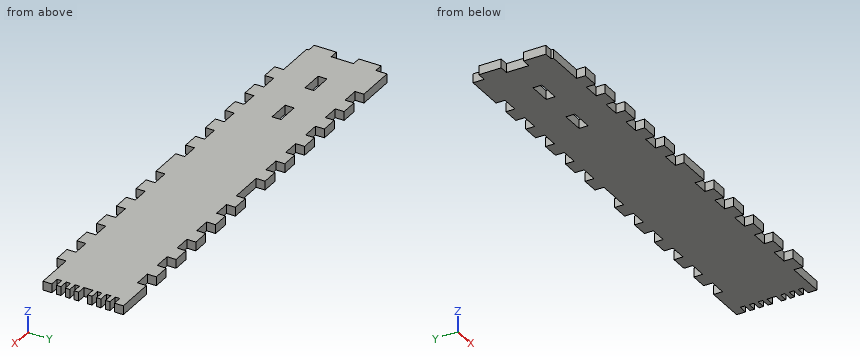
from build123d import *

# Parameters (mm, degrees)
ESQUISSE1_W             = 400
ESQUISSE1_H             = 80
BOSS_EXTRU_1_DEPTH      = 8
ESQUISSE2_W             = 8
ESQUISSE2_H             = 20
BOSS_EXTRU_2_DEPTH      = 8
ESQUISSE4_W             = 15
ESQUISSE4_H             = 8
ENL_V_MAT_EXTRU_1_DEPTH = 212.962260792
ESQUISSE5_W             = 15
ESQUISSE5_H             = 8
ESQUISSE5_W_2           = 35
ENL_V_MAT_EXTRU_2_DEPTH = 212.962260792
ESQUISSE6_W             = 20
ESQUISSE6_H             = 8
ENL_V_MAT_EXTRU_3_DEPTH = 212.962260792
ESQUISSE8_W             = 8
ESQUISSE8_H             = 4
ENL_V_MAT_EXTRU_5_DEPTH = 212.962260792


with BuildPart() as part:
    # Esquisse1 → Boss.-Extru.1 (new body)
    with BuildSketch(Plane.XY):
        Rectangle(ESQUISSE1_W, ESQUISSE1_H)
    extrude(amount=BOSS_EXTRU_1_DEPTH)

    # Esquisse2 → Boss.-Extru.2 (add)
    with BuildSketch(Plane.XY):
        with Locations((-204, 20)):
            Rectangle(ESQUISSE2_W, ESQUISSE2_H)
        with Locations((-204, -20)):
            Rectangle(ESQUISSE2_W, ESQUISSE2_H)
    extrude(amount=BOSS_EXTRU_2_DEPTH)

    # Esquisse4 → Enlèv. mat.-Extru.1 (cut, through all)
    with BuildSketch(Plane.XY):
        Polygon((0, 40), (-15, 40), (-15, 32), (0, 32), (15, 32), (15, 40), align=None)
        with Locations((-37.5, 36)):
            Rectangle(ESQUISSE4_W, ESQUISSE4_H)
        with Locations((-67.5, 36)):
            Rectangle(ESQUISSE4_W, ESQUISSE4_H)
        with Locations((-97.5, 36)):
            Rectangle(ESQUISSE4_W, ESQUISSE4_H)
        with Locations((-127.5, 36)):
            Rectangle(ESQUISSE4_W, ESQUISSE4_H)
        with Locations((-157.5, 36)):
            Rectangle(ESQUISSE4_W, ESQUISSE4_H)
        with Locations((37.5, 36)):
            Rectangle(ESQUISSE4_W, ESQUISSE4_H)
        with Locations((67.5, 36)):
            Rectangle(ESQUISSE4_W, ESQUISSE4_H)
        with Locations((97.5, 36)):
            Rectangle(ESQUISSE4_W, ESQUISSE4_H)
        with Locations((127.5, 36)):
            Rectangle(ESQUISSE4_W, ESQUISSE4_H)
        with Locations((157.5, 36)):
            Rectangle(ESQUISSE4_W, ESQUISSE4_H)
    extrude(amount=ENL_V_MAT_EXTRU_1_DEPTH, mode=Mode.SUBTRACT)

    # Esquisse5 → Enlèv. mat.-Extru.2 (cut, through all)
    with BuildSketch(Plane.XY):
        with Locations((-22.5, -36)):
            Rectangle(ESQUISSE5_W, ESQUISSE5_H)
        with Locations((-52.5, -36)):
            Rectangle(ESQUISSE5_W, ESQUISSE5_H)
        with Locations((-82.5, -36)):
            Rectangle(ESQUISSE5_W, ESQUISSE5_H)
        with Locations((-112.5, -36)):
            Rectangle(ESQUISSE5_W, ESQUISSE5_H)
        with Locations((-142.5, -36)):
            Rectangle(ESQUISSE5_W, ESQUISSE5_H)
        with Locations((-182.5, -36)):
            Rectangle(ESQUISSE5_W_2, ESQUISSE5_H)
        with Locations((22.5, -36)):
            Rectangle(ESQUISSE5_W, ESQUISSE5_H)
        with Locations((52.5, -36)):
            Rectangle(ESQUISSE5_W, ESQUISSE5_H)
        with Locations((82.5, -36)):
            Rectangle(ESQUISSE5_W, ESQUISSE5_H)
        with Locations((112.5, -36)):
            Rectangle(ESQUISSE5_W, ESQUISSE5_H)
        with Locations((142.5, -36)):
            Rectangle(ESQUISSE5_W, ESQUISSE5_H)
        with Locations((182.5, -36)):
            Rectangle(ESQUISSE5_W_2, ESQUISSE5_H)
    extrude(amount=ENL_V_MAT_EXTRU_2_DEPTH, mode=Mode.SUBTRACT)

    # Esquisse6 → Enlèv. mat.-Extru.3 (cut, through all)
    with BuildSketch(Plane.XY):
        with Locations((-160, 0)):
            Rectangle(ESQUISSE6_W, ESQUISSE6_H)
        with Locations((-110, 0)):
            Rectangle(ESQUISSE6_W, ESQUISSE6_H)
    extrude(amount=ENL_V_MAT_EXTRU_3_DEPTH, mode=Mode.SUBTRACT)

    # Esquisse8 → Enlèv. mat.-Extru.5 (cut, through all)
    with BuildSketch(Plane.XY):
        Polygon((200, 4), (200, 8), (192, 8), (192, 4), (192, 0), (200, 0), align=None)
        with Locations((196, 14)):
            Rectangle(ESQUISSE8_W, ESQUISSE8_H)
        with Locations((196, 22)):
            Rectangle(ESQUISSE8_W, ESQUISSE8_H)
        with Locations((196, 30)):
            Rectangle(ESQUISSE8_W, ESQUISSE8_H)
        with Locations((196, -6)):
            Rectangle(ESQUISSE8_W, ESQUISSE8_H)
        with Locations((196, -14)):
            Rectangle(ESQUISSE8_W, ESQUISSE8_H)
        with Locations((196, -22)):
            Rectangle(ESQUISSE8_W, ESQUISSE8_H)
    extrude(amount=ENL_V_MAT_EXTRU_5_DEPTH, mode=Mode.SUBTRACT)


solid = part.part
Model file for the job. Use its own axes, mm. Give positions to 0.01 mm unless a question says otherwise; leave off trailing zeros. Loops run counter-clockwise (first coordinate to the right, second up) from the corner with the lowest first, then second, coordinate; pieces in that order, holes last. Notation, with made-up numbers: (89.5, -5.75) - (145.5, -5.75) arc R22 cw to (145.5, 18.25) - close; hole circle Ø3 at (-19, -7). An arc over 180 degrees is marked (long way). Use one line per item in the form item = value.
(1) Cut at B-B (z = 6). Count the separate pieces of the cut face and the enclosed holes in it, then the cut area to 3 significant figures.
Determined:
separate_pieces = 1
enclosed_holes = 2
area = 28,500 mm^2
(2) Drill centre lines: L1, parallel to X at y = 5, z = 1; L2, parallel to Y at x = 27, z = 5; L3, parallel to Y at x = -157, z = 7.75. Where is each one in solid material? Low to high.
Determined:
L1 = -200 to 192
L2 = -32 to 40
L3 = -40 to -4, 4 to 32
(3) Drop flat-ended pins along their axis: P1, Ø1, axis at x = -129, z = 6, coming from the +Y side; P2, Ø1.5, axis at x = 112, z = 6, coming from the -Y side; P3, Ø3, axis at y = 5.5, z = 5.5, coming from the +X side; P4, Ø5, axis at x = 73, y = -22, coming from the -Z side. Give the stop position or say it passes through.
Determined:
P1 = 32
P2 = -32
P3 = 192
P4 = 0
(4) Cut at A-A (x = -158). Give the cut face in (y, z), then the cut area to 3 significant figures.
Determined:
outline = (-40, 0) - (-4, 0) - (-4, 8) - (-40, 8) - close; (4, 0) - (32, 0) - (32, 8) - (4, 8) - close
area = 512 mm^2
